Could you check a few things on this model? Use its own coordinates, in mm. Face numbers are marked on the shaded views. A direction names the side the tool comes from. Give positions to 0.01 mm unless a question says otherwise; leave off trailing zeros. Write each loop counter-clockwise with the first axis right and the second up, starting at its lowest first coordinate (ties: lowest second). Pieces come first, ordered by that corner, then holes. Notation, with made-up numbers: (86.5, 42) - (100.5, 42) arc R20 ccw to (100.5, 52) - close; hole circle Ø8 at (62, 52.5). An arc over 180 degrees is marked (long way). Use one line per item in the form item = value.
```python
from build123d import *

# Parameters (mm, degrees)
F1_DEPTH       = 20
F3_D           = 4.5
F3_CSINK_D     = 8
F3_CSINK_ANGLE = 90


with BuildPart() as f1:
    # F0 (on Right) → F1 (new body, symmetric)
    with BuildSketch(Plane.YZ):
        with BuildLine():
            ThreePointArc((26.95, 0), (25.778427, 2.828427), (22.95, 4))
            Line((22.95, 4), (-17.95, 4))
            Line((-17.95, 4), (-17.95, 17))
            Line((-17.95, 17), (7.05, 17))
            ThreePointArc((7.05, 17), (5.878427, 19.828427), (3.05, 21))
            Line((3.05, 21), (-18.790565, 21))
            ThreePointArc((-18.790565, 21), (-21.269887, 20.138943), (-22.68179, 17.926482))
            Line((-22.68179, 17.926482), (-26.95, 0))
            Line((-26.95, 0), (26.95, 0))
        make_face()
    extrude(amount=F1_DEPTH, both=True)

    # F3 (through all)
    with Locations(Plane.XY.offset(4)):
        with Locations((-10, 12.870283), (10, 12.870283)):
            CounterSinkHole(F3_D / 2, F3_CSINK_D / 2, counter_sink_angle=F3_CSINK_ANGLE)


solid = f1.part
```
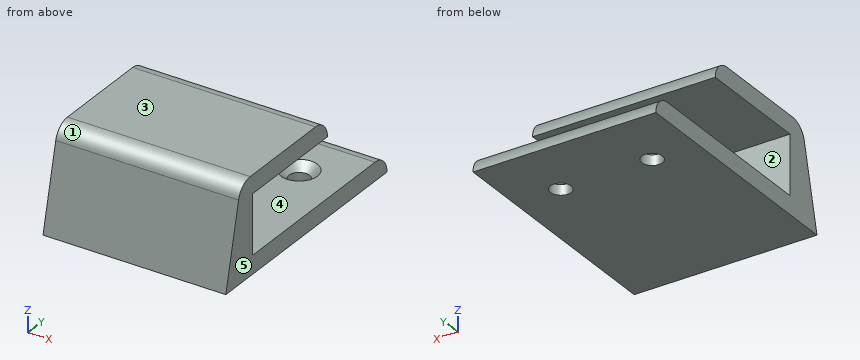
1. For pin 1 (12 mm diameter, centred on x = 15.5, y = 21, fed in from +Z); pin 2 (2 mm diameter, centred on x = -1, z = 14.5, fed in from -Y); pin 3 (10.5 mm diameter, centred on x = 2, z = 12.5, fed in from +Y); pin 4 (3 mm diameter, centred on y = -15, z = 11.5, fed in from -X), each with a flat end and sliding along its axis, tell me the tip position at first contact or that it passes through.
Response values:
pin_1 = 4
pin_2 = -23.74
pin_3 = 7.05
pin_4 = through
2. Which directions (+Z, -Z, +X, -X, +Y, -Y) give clear straight access to the entire face, cutting with the end or side of a thin tool? Please do the marked faces 1 and 2.
Response values:
face_1 = +Z, +X, -X, -Y
face_2 = +X, -X, +Y
3. Imagine slicing it at B-B, the plane x = 10. List the corners of the cut face in (y, z) for me, and give its area (3 significant figures).
Response values:
outline = (-26.95, 0) - (10.62, 0) - (10.62, 2.25) - (8.87, 4) - (-17.95, 4) - (-17.95, 17) - (7.05, 17) arc R4 ccw to (3.05, 21) - (-18.79, 21) arc R4 ccw to (-22.68, 17.93) - close; (15.12, 0) - (26.95, 0) arc R4 ccw to (22.95, 4) - (16.87, 4) - (15.12, 2.25) - close
area = 386 mm²
4. If we mould it in two halves opening along Z, with no side actions, what happens to the marked faces 3, 4 and 5? For each: pulls with the +Z half, pulls with the -Z half, needs draft (parallel to the pull), parting line crosses it, or undercut.
Response values:
face_3 = pulls with the +Z half
face_4 = undercut
face_5 = needs draft
5. If I drill on line 1 (Z direction, x = 11, y = -7); line 2 (Y direction, x = 10, z = 0.8); line 3 (Z direction, x = -3.5, y = 6.5), over which ranges is the centre line in solid material (lowest first)? Write a range as from..to.
Response values:
line_1 = 0..4, 17..21
line_2 = -26.76..10.62, 15.12..26.87
line_3 = 0..4, 17..19.02
6. Imagine slicing it at D-D, the plane z = 3. List the corners of the cut face in (x, y) for me.
Response values:
outline = (-20, -26.24) - (20, -26.24) - (20, 25.6) - (-20, 25.6) - close; hole circle Ø6 at (-10, 12.87); hole circle Ø6 at (10, 12.87)
7. Imagine slicing it at C-C, the plane x = -15. List the corners of the cut face in (y, z) for me, and give its area (3 significant figures).
Response values:
outline = (-26.95, 0) - (26.95, 0) arc R4 ccw to (22.95, 4) - (-17.95, 4) - (-17.95, 17) - (7.05, 17) arc R4 ccw to (3.05, 21) - (-18.79, 21) arc R4 ccw to (-22.68, 17.93) - close
area = 407 mm²
8. Imagine slicing it at A-A, the plane y = -14.5. List the corners of the cut face in (x, z) for me.
Response values:
outline = (-20, 0) - (20, 0) - (20, 4) - (-20, 4) - close; (-20, 17) - (20, 17) - (20, 21) - (-20, 21) - close
